Here's how the part is built. I have some questions about the finished solid (model axes, mm). A direction names the side the tool comes from. Round coordinates to 2 decimals unless told otherwise and drop trailing zeros. Write each loop counter-clockwise with the first axis right and the second up, starting at its lowest first coordinate (ties: lowest second). Pieces come first, ordered by that corner, then holes. Notation, with made-up numbers: (26, -32.5) -> (46, -32.5) arc R18 cw to (46, -18.5) -> close; hole circle Ø9 at (31.5, 33.25). An arc over 180 degrees is marked (long way). Put each result on its own line as item: value. Start each with the question number.
1. For pin 1 (7.5 mm diameter, centred on y = 219.5, z = 848.5, fed in from +X); pin 2 (15 mm diameter, centred on x = -100, z = 14.5, fed in from -Y); pin 3 (12 mm diameter, centred on x = -170.5, y = 18.5, fed in from +Z), each with a flat end and sliding along its axis, tell me the tip position at first contact or that it passes through.
2. Suppose I cut it at D-D (y = 67.5). Please give me the cut outline in (x, z).
3. We'd pull the mould along Y, two halves only. Please class faces 1 (the face through (300, -3, 25)), 2 (the face through (-275, -250, 25)), 3 (the face through (-25.4, 111, 25)): +Y half, -Y half, draft (parallel to the pull), parting line (faces both ways), or undercut.
4. I need wall thicknesses on probe 1 along Z at (x, y) = (-32.5, -21.5); probe 2 along Y at (x, z) = (-20, 164.5); probe 3 along Z at (x, y) = (270, 58.5). Which ranges of each line are inside material? Lowest first, please. Write a range as from..to.
5. Suppose I cut it at B-B (z = 497.5). Please give me the cut outline in (x, y), then the cut area to 3 significant figures.
6. Suppose I cut it at C-C (x = 126). Please give me the cut outline in (y, z).
7. Suppose I cut it at A-A (x = 61). Please give me the cut outline in (y, z), then the cut area to 3 significant figures.
8. Which directions (+Z, -Z, +X, -X, +Y, -Y) give clear straight access to the entire face, cutting with the end or side of a thin tool? Please do faces 4 (the face through (-25.4, 0, 421)), 5 (the face through (-20, -25.4, 302)), 6 (the face through (252, 59, 50.8)), 7 (the face through (-103, 4, 851)), 8 (the face through (-20, 25.4, 280)).
```python
from build123d import *

# Parameters (mm, degrees)
F0_W     = 223.8
F0_H     = 173.8
F1_DEPTH = 50.8
F2_W     = 51.225417
F2_H     = 50.8
F2_W_2   = 50.8
F3_DEPTH = 750
F5_W     = 76.2
F5_H     = 275.4
F6_DEPTH = 38.1
F8_W     = 206
F8_H     = 60
F9_DEPTH = 25.4


with BuildPart() as f1:
    # F0 (on Top) → F1 (new body)
    with BuildSketch(Plane.XY):
        Polygon((0, 250), (-300, 250), (-300, -250), (-249.2, -250), (-249.2, -25.4), (0, -25.4), (249.2, -25.4), (249.2, -250), (300, -250), (300, 250), align=None)
        with Locations((-137.3, 112.3)):
            Rectangle(F0_W, F0_H, mode=Mode.SUBTRACT)
        with Locations((137.3, 112.3)):
            Rectangle(F0_W, F0_H, mode=Mode.SUBTRACT)
    extrude(amount=F1_DEPTH)

    # F2 (on face) → F3 (join)
    with BuildSketch(Plane.XY.offset(50.8)):
        with Locations((0.212708, 0)):
            Rectangle(F2_W, F2_H)
        with Locations((0, 224.6)):
            Rectangle(F2_W_2, F2_H)
    extrude(amount=F3_DEPTH)

    # F5 (on offset) → F6 (join)
    with BuildSketch(Plane.XY.offset(800.8)):
        with Locations((0, 112.3)):
            Rectangle(F5_W, F5_H)
    extrude(amount=F6_DEPTH)

    # F8 (on offset) → F9 (join)
    with BuildSketch(Plane.XY.offset(838.9)):
        with Locations((0, 4.6)):
            Rectangle(F8_W, F8_H)
        with Locations((0, 220)):
            Rectangle(F8_W, F8_H)
    extrude(amount=F9_DEPTH)


solid = f1.part
```
Verdict:
1. pin 1: stops at x = 103
1. pin 2: stops at y = -25.4
1. pin 3: stops at z = 50.8
2. outline: (-300, 0) -> (-249.2, 0) -> (-249.2, 50.8) -> (-300, 50.8) -> close; (-38.1, 800.8) -> (38.1, 800.8) -> (38.1, 838.9) -> (-38.1, 838.9) -> close; (-25.4, 0) -> (25.4, 0) -> (25.4, 50.8) -> (-25.4, 50.8) -> close; (249.2, 0) -> (300, 0) -> (300, 50.8) -> (249.2, 50.8) -> close
3. face 1: draft
3. face 2: -Y half
3. face 3: undercut
4. probe 1: z = 0..50.8, 800.8..864.3
4. probe 2: y = -25.4..25.4, 199.2..250
4. probe 3: z = 0..50.8
5. outline: (-25.4, -25.4) -> (25.83, -25.4) -> (25.83, 25.4) -> (-25.4, 25.4) -> close; (-25.4, 199.2) -> (25.4, 199.2) -> (25.4, 250) -> (-25.4, 250) -> close
5. area: 5,180 mm^2
6. outline: (-25.4, 0) -> (25.4, 0) -> (25.4, 50.8) -> (-25.4, 50.8) -> close; (199.2, 0) -> (250, 0) -> (250, 50.8) -> (199.2, 50.8) -> close
7. outline: (-25.4, 0) -> (25.4, 0) -> (25.4, 50.8) -> (-25.4, 50.8) -> close; (-25.4, 838.9) -> (34.6, 838.9) -> (34.6, 864.3) -> (-25.4, 864.3) -> close; (190, 838.9) -> (250, 838.9) -> (250, 864.3) -> (190, 864.3) -> close; (199.2, 0) -> (250, 0) -> (250, 50.8) -> (199.2, 50.8) -> close
7. area: 8,210 mm^2
8. face 4: -X, +Y, -Y
8. face 5: +Z, -Z, -Y
8. face 6: +X, +Y, -Y
8. face 7: +Z, -X, +Y, -Y
8. face 8: none
